Could you check a few things on this model? Use its own coordinates, in mm. A direction names the side the tool comes from. Give positions to 0.01 mm unless a question says otherwise; leave off trailing zeros. Write each loop counter-clockwise with the first axis right and the second up, starting at its lowest first coordinate (ties: lowest second). Pieces come first, ordered by that corner, then holes. Notation, with made-up numbers: (23.25, 68) - (78.25, 68) arc R21 ccw to (78.25, 96) - close; hole circle Ø6 at (3.5, -28). An arc over 180 degrees is marked (long way). Answer in a Markdown table with one row per item.
from build123d import *

# Parameters (mm, degrees)
SKETCH_1_R      = 2.5
EXTRUDE_1_DEPTH = 6


with BuildPart() as part:
    # Эскиз1 → Бобышка-Вытянуть1 (new body)
    with BuildSketch(Plane.XY):
        with BuildLine():
            Line((-28, -30.6), (-27.75, -24.6))
            Line((-27.75, -24.6), (27.75, -24.6))
            Line((27.75, -24.6), (28, -30.6))
            Line((28, -30.6), (38, -30.6))
            Line((38, -30.6), (38.25, -24.6))
            Line((38.25, -24.6), (55.95, -24.6))
            Line((55.95, -24.6), (55.95, -17.8))
            Line((55.95, -17.8), (54.75, -17.8))
            Line((54.75, -17.8), (54.75, -15.6))
            Line((54.75, -15.6), (55.95, -15.6))
            Line((55.95, -15.6), (55.95, -14.1))
            Line((55.95, -14.1), (59.05, -14.1))
            Line((59.05, -14.1), (59.05, -15.6))
            Line((59.05, -15.6), (60.25, -15.6))
            Line((60.25, -15.6), (60.25, -17.8))
            Line((60.25, -17.8), (59.05, -17.8))
            Line((59.05, -17.8), (59.05, -24.6))
            Line((59.05, -24.6), (71.55, -24.6))
            Line((71.55, -24.6), (76.75, -24.6))
            Line((76.75, -24.6), (77, -30.6))
            Line((77, -30.6), (87, -30.6))
            Line((87, -30.6), (87.25, -24.6))
            Line((87.25, -24.6), (126.5, -24.6))
            Line((126.5, -24.6), (126.5, -18.65))
            Line((126.5, -18.65), (132.5, -18.6))
            Line((132.5, -18.6), (132.5, -8.6))
            Line((132.5, -8.6), (126.5, -8.55))
            Line((126.5, -8.55), (126.5, -6.15))
            Line((126.5, -6.15), (119.7, -6.15))
            Line((119.7, -6.15), (119.7, -7.35))
            Line((119.7, -7.35), (117.5, -7.35))
            Line((117.5, -7.35), (117.5, -6.15))
            Line((117.5, -6.15), (116, -6.15))
            Line((116, -6.15), (116, -3.05))
            Line((116, -3.05), (117.5, -3.05))
            Line((117.5, -3.05), (117.5, -1.85))
            Line((117.5, -1.85), (119.7, -1.85))
            Line((119.7, -1.85), (119.7, -3.05))
            Line((119.7, -3.05), (126.5, -3.05))
            Line((126.5, -3.05), (126.5, -0.65))
            Line((126.5, -0.65), (132.5, -0.6))
            Line((132.5, -0.6), (132.5, 9.4))
            Line((132.5, 9.4), (126.5, 9.45))
            Line((126.5, 9.45), (94.5, 9.45))
            ThreePointArc((94.5, 9.45), (92.378679656, 10.328679656), (91.5, 12.45))
            Line((91.5, 12.45), (91.5, 15.4))
            Line((91.5, 15.4), (87.25, 15.4))
            Line((87.25, 15.4), (87, 21.4))
            Line((87, 21.4), (77, 21.4))
            Line((77, 21.4), (76.75, 15.4))
            Line((76.75, 15.4), (59.05, 15.4))
            Line((59.05, 15.4), (59.05, 8.6))
            Line((59.05, 8.6), (60.25, 8.6))
            Line((60.25, 8.6), (60.25, 6.4))
            Line((60.25, 6.4), (59.05, 6.4))
            Line((59.05, 6.4), (59.05, 4.9))
            Line((59.05, 4.9), (55.95, 4.9))
            Line((55.95, 4.9), (55.95, 6.4))
            Line((55.95, 6.4), (54.75, 6.4))
            Line((54.75, 6.4), (54.75, 8.6))
            Line((54.75, 8.6), (55.95, 8.6))
            Line((55.95, 8.6), (55.95, 15.4))
            Line((55.95, 15.4), (38.25, 15.4))
            Line((38.25, 15.4), (38, 21.4))
            Line((38, 21.4), (38, 25.4))
            Line((38, 25.4), (37.942164229, 25.4))
            Line((37.942164229, 25.4), (37.942164229, 29.6))
            ThreePointArc((37.942164229, 29.6), (36.942164229, 30.6), (35.942164229, 29.6))
            Line((35.942164229, 29.6), (35.942164229, 26))
            ThreePointArc((35.942164229, 26), (35.766428298, 25.575735931), (35.342164229, 25.4))
            Line((35.342164229, 25.4), (28.5, 25.4))
            ThreePointArc((28.5, 25.4), (28.146446609, 25.253553391), (28, 24.9))
            Line((28, 24.9), (28, 21.4))
            Line((28, 21.4), (27.75, 15.4))
            Line((27.75, 15.4), (-27.75, 15.4))
            Line((-27.75, 15.4), (-28, 21.4))
            Line((-28, 21.4), (-38, 21.4))
            Line((-38, 21.4), (-38.25, 15.4))
            Line((-38.25, 15.4), (-43.45, 15.4))
            Line((-43.45, 15.4), (-55.95, 15.4))
            Line((-55.95, 15.4), (-55.95, 8.6))
            Line((-55.95, 8.6), (-54.75, 8.6))
            Line((-54.75, 8.6), (-54.75, 6.4))
            Line((-54.75, 6.4), (-55.95, 6.4))
            Line((-55.95, 6.4), (-55.95, 4.9))
            Line((-55.95, 4.9), (-59.05, 4.9))
            Line((-59.05, 4.9), (-59.05, 6.4))
            Line((-59.05, 6.4), (-60.25, 6.4))
            Line((-60.25, 6.4), (-60.25, 8.6))
            Line((-60.25, 8.6), (-59.05, 8.6))
            Line((-59.05, 8.6), (-59.05, 15.4))
            Line((-59.05, 15.4), (-64.25, 15.4))
            Line((-64.25, 15.4), (-76.75, 15.4))
            Line((-76.75, 15.4), (-77, 21.4))
            Line((-77, 21.4), (-87, 21.4))
            Line((-87, 21.4), (-87.25, 15.4))
            Line((-87.25, 15.4), (-91.5, 15.4))
            Line((-91.5, 15.4), (-91.5, 12.45))
            ThreePointArc((-91.5, 12.45), (-92.378679656, 10.328679656), (-94.5, 9.45))
            Line((-94.5, 9.45), (-126.5, 9.45))
            Line((-126.5, 9.45), (-132.5, 9.4))
            Line((-132.5, 9.4), (-132.5, -0.6))
            Line((-132.5, -0.6), (-126.5, -0.65))
            Line((-126.5, -0.65), (-126.5, -3.05))
            Line((-126.5, -3.05), (-119.7, -3.05))
            Line((-119.7, -3.05), (-119.7, -1.85))
            Line((-119.7, -1.85), (-117.5, -1.85))
            Line((-117.5, -1.85), (-117.5, -3.05))
            Line((-117.5, -3.05), (-116, -3.05))
            Line((-116, -3.05), (-116, -6.15))
            Line((-116, -6.15), (-117.5, -6.15))
            Line((-117.5, -6.15), (-117.5, -7.35))
            Line((-117.5, -7.35), (-119.7, -7.35))
            Line((-119.7, -7.35), (-119.7, -6.15))
            Line((-119.7, -6.15), (-126.5, -6.15))
            Line((-126.5, -6.15), (-126.5, -8.55))
            Line((-126.5, -8.55), (-132.5, -8.6))
            Line((-132.5, -8.6), (-132.5, -18.6))
            Line((-132.5, -18.6), (-126.5, -18.65))
            Line((-126.5, -18.65), (-126.5, -24.6))
            Line((-126.5, -24.6), (-87.25, -24.6))
            Line((-87.25, -24.6), (-87, -30.6))
            Line((-87, -30.6), (-77, -30.6))
            Line((-77, -30.6), (-76.75, -24.6))
            Line((-76.75, -24.6), (-64.25, -24.6))
            Line((-64.25, -24.6), (-59.05, -24.6))
            Line((-59.05, -24.6), (-59.05, -17.8))
            Line((-59.05, -17.8), (-60.25, -17.8))
            Line((-60.25, -17.8), (-60.25, -15.6))
            Line((-60.25, -15.6), (-59.05, -15.6))
            Line((-59.05, -15.6), (-59.05, -14.1))
            Line((-59.05, -14.1), (-55.95, -14.1))
            Line((-55.95, -14.1), (-55.95, -15.6))
            Line((-55.95, -15.6), (-54.75, -15.6))
            Line((-54.75, -15.6), (-54.75, -17.8))
            Line((-54.75, -17.8), (-55.95, -17.8))
            Line((-55.95, -17.8), (-55.95, -24.6))
            Line((-55.95, -24.6), (-43.45, -24.6))
            Line((-43.45, -24.6), (-38.25, -24.6))
            Line((-38.25, -24.6), (-38, -30.6))
            Line((-38, -30.6), (-28, -30.6))
        make_face()
        with Locations((0, -14.6)):
            Circle(SKETCH_1_R, mode=Mode.SUBTRACT)
        with Locations((0, 5.4)):
            Circle(SKETCH_1_R, mode=Mode.SUBTRACT)
    extrude(amount=EXTRUDE_1_DEPTH)


solid = part.part
1) Imagine slicing it at C-C (z = 1.7). State how many separate pieces and enclosed holes the cut face has, then the cut area to 3 significant figures.
Check values:
| item | result |
|---|---|
| separate pieces | 1 |
| enclosed holes | 2 |
| area | 10,200 mm2 |
2) Imagine slicing it at B-B (x = -83). List the corners of the cut face in (y, z) for me.
Check values:
| item | result |
|---|---|
| outline | (-30.6, 0) - (21.4, 0) - (21.4, 6) - (-30.6, 6) - close |
3) If I drill on line 1 (Y direction, x = 0, z = 1.9); line 2 (Y direction, x = -55.5, z = 3.05); line 3 (X direction, y = 6, z = 0.9), over which ranges is the centre line in solid material (lowest first)?
Check values:
| item | result |
|---|---|
| line 1 | y = -24.6 to -17.1, -12.1 to 2.9, 7.9 to 15.4 |
| line 2 | y = -24.6 to -17.8, -15.6 to 6.4, 8.6 to 15.4 |
| line 3 | x = -132.5 to -59.05, -55.95 to -2.43, 2.43 to 55.95, 59.05 to 132.5 |
4) We'd pull the mould along X, two halves only. Please class faces 1 (the face through (111, 9.45, 3)), 2 (the face through (-55.95, 12, 3)): +X half, -X half, draft (parallel to the pull), parting line (faces both ways), or undercut.
Check values:
| item | result |
|---|---|
| face 1 | draft |
| face 2 | undercut |
5) Will these pins go through, and if not, where does the flat tip stop? P1, Ø1.1, axis at y = 27.5, z = 2, coming from the -X side; P2, Ø3, axis at x = -46, z = 3.5, coming from the +Y side; P3, Ø1.8, axis at y = 24, z = 4, coming from the -X side.
Check values:
| item | result |
|---|---|
| P1 | stops at x = 35.94 |
| P2 | stops at y = 15.4 |
| P3 | stops at x = 28 |
6) On a 3-axis mill with a long thin cutter (end or side, diameter ignored), from which of +Z, -Z, +X, -X, +Y, -Y can I reach the whole of each face in a straight line? I mean faces 3 (the face through (-59.05, 12, 3)), 4 (the face through (-123, -6.15, 3)), 5 (the face through (0, -24.6, 3)). Say none if no direction works.
Check values:
| item | result |
|---|---|
| face 3 | +Z, -Z, +Y |
| face 4 | +Z, -Z, -X |
| face 5 | +Z, -Z, -Y |
7) Imagine slicing it at D-D (x = 32). List the corners of the cut face in (y, z) for me.
Check values:
| item | result |
|---|---|
| outline | (-30.6, 0) - (25.4, 0) - (25.4, 6) - (-30.6, 6) - close |
8) Imagine slicing it at A-A (x = 0). List the corners of the cut face in (y, z) for me, then the cut area to 3 significant figures.
Check values:
| item | result |
|---|---|
| outline | (-24.6, 0) - (-17.1, 0) - (-17.1, 6) - (-24.6, 6) - close; (-12.1, 0) - (2.9, 0) - (2.9, 6) - (-12.1, 6) - close; (7.9, 0) - (15.4, 0) - (15.4, 6) - (7.9, 6) - close |
| area | 180 mm2 |
